Can you work these out from the drawing? Everything is in mm from the part's minimum corner. A direction names the side the tool comes from. Coordinates: 2 decimals unless noted, no trailing zeros. Write each loop counter-clockwise with the first axis right and the second up, starting at its lowest first coordinate (ties: lowest second). Pieces come first, ordered by that corner, then holes. Notation, with made-up numbers: M 27,25 L 67,25 A18 ccw 67,53 Z; hole C 56,-20 d7. An arc over 180 degrees is marked long. Use one line per item in the form item = value. Start each with the question number.
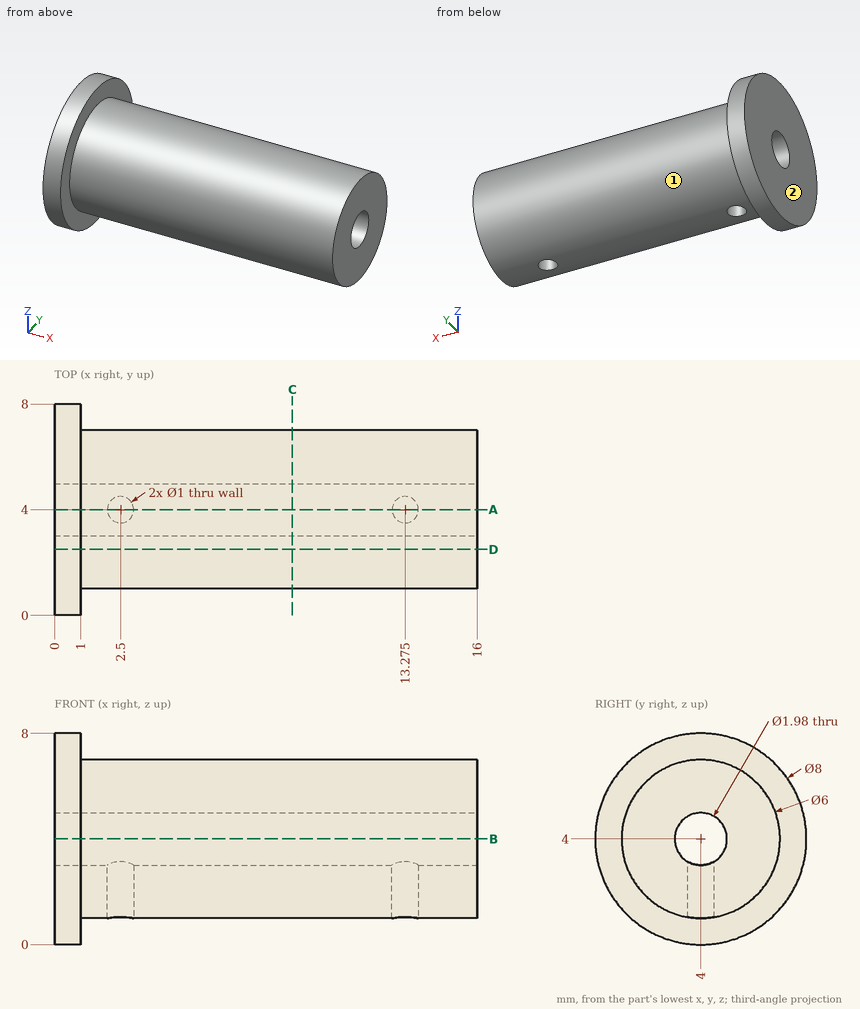
1) Will these pins go through, and if not, where does the flat tip stop? pin 1 Ø4 at (x, y) = (2, 2.5) entering from -Z; pin 2 Ø1.5 at (x, z) = (13, 2.5) entering from -Y (1 decimal).
2) Suppose I cut it at D-D on y = 2.5. Please give me the cut outline in (x, z).
3) Please list where these lines run through material, in increasing order: line 1 (X direction, y = 4, z = 2.7) (3 decimals); line 2 (Y direction, x = 11.75, z = 4).
4) Which directions (+Z, -Z, +X, -X, +Y, -Y) give clear straight access to the entire face, cutting with the end or side of a thin tool? Please do the marked faces 1 and 2.
5) Suppose I cut it at A-A on y = 4. Please give me the cut outline in (x, z) (3 decimals), and give its area (3 significant figures).
6) Suppose I cut it at C-C on x = 9. Please give me the cut outline in (y, z), and give its area (3 significant figures).
7) Suppose I cut it at B-B on z = 4. Please give me the cut outline in (x, y), and give its area (3 significant figures).
Computed values:
q1.pin_1 = 0
q1.pin_2 = 1.1
q2.outline = M 0,0.29 L 1,0.29 L 1,1.4 L 16,1.4 L 16,6.6 L 1,6.6 L 1,7.71 L 0,7.71 Z
q3.line_1 = 0 to 2, 3 to 12.775, 13.775 to 16
q3.line_2 = 1 to 3.01, 4.99 to 7
q4.face_1 = +X
q4.face_2 = +Z, -Z, -X, +Y, -Y
q5.outline = M 0,0 L 1,0 L 1,1 L 2,1 L 2,3.01 L 0,3.01 Z; M 0,4.99 L 16,4.99 L 16,7 L 1,7 L 1,8 L 0,8 Z; M 3,1 L 12.775,1 L 12.775,3.01 L 3,3.01 Z; M 13.775,1 L 16,1 L 16,3.01 L 13.775,3.01 Z
q5.area = 62.3 mm²
q6.outline = C 4,4 d6; hole C 4,4 d1.98
q6.area = 25.2 mm²
q7.outline = M 0,0 L 1,0 L 1,1 L 16,1 L 16,3.01 L 0,3.01 Z; M 0,4.99 L 16,4.99 L 16,7 L 1,7 L 1,8 L 0,8 Z
q7.area = 66.3 mm²
